Could you check a few things on this model? Use its own coordinates, in mm. A direction names the side the tool comes from. Coordinates: 2 decimals unless noted, no trailing zeros. Loops run counter-clockwise (first coordinate to the right, second up) from the corner with the lowest first, then second, coordinate; pieces in that order, holes last. Notation, with made-up numbers: M -35,-17 L -15,-17 A17 ccw -15,-9 Z; hole C 62.25,-32.5 d4. An arc over 180 degrees is marked long. Write each question's results on one line, items separated by ' | '.
```python
from build123d import *

# Parameters (mm, degrees)
F0_R     = 12.7
F1_DEPTH = 25.4
F2_R     = 15.875
F2_R_2   = 12.7
F3_DEPTH = 3.175


with BuildPart() as f1:
    # F0 (on Front) → F1 (new body)
    with BuildSketch(Plane.XZ):
        Circle(F0_R)
        with BuildLine():
            ThreePointArc((-1.8139228208, -1.778), (-0.9602697629, 2.351485059), (2.54, 0))
            ThreePointArc((2.54, 0), (2.351485059, -0.9602697629), (1.8139228208, -1.778))
            ThreePointArc((1.8139228208, -1.778), (0, -2.54), (-1.8139228208, -1.778))
        make_face(mode=Mode.SUBTRACT)
        with BuildLine():
            Line((1.8139228208, -1.778), (-1.8139228208, -1.778))
            ThreePointArc((-1.8139228208, -1.778), (0, -2.54), (1.8139228208, -1.778))
        make_face()
    extrude(amount=F1_DEPTH)

    # F2 (on face) → F3 (join)
    with BuildSketch(Plane.XZ.offset(25.4)):
        Circle(F2_R)
        Circle(F2_R_2, mode=Mode.SUBTRACT)
    extrude(amount=-F3_DEPTH)

    # F5: F1 across plane


with BuildPart() as f1_1:
    add(f1.part)
    add(f1.part.mirror(Plane(origin=(0, -12.7, -0.0066463366), x_dir=(1, 0, 0), z_dir=(0, 1, 0))))


solid = f1_1.part
```
(1) If we mould it in two halves opening along Y, with no side actions, what happens to faces 3 (the flat face through (3, 0, 0)), 4 (the flat face through (0, -13, -1.778)), 5 (the flat face through (-7, -3.175, 11))? For each: released by +Y, released by -Y, zero draft, split by the parting line, or undercut.
Reported:
face 3: released by +Y | face 4: zero draft | face 5: undercut
(2) Which directions (+Z, -Z, +X, -X, +Y, -Y) give clear straight access to the entire face, cutting with the end or side of a thin tool? Please do faces 1 (the cylindrical face through (-2.75, -12.57, -12.4)), 2 (the cylindrical face through (-3.441, -23.835, -15.497)).
Reported:
face 1: none | face 2: +Y, -Y
(3) Imagine slicing it at D-D, the plane z = -3. List the corners of the cut face in (x, y) for me (3 decimals), and give its area (3 significant figures).
Reported:
outline: M -15.589,-25.4 L 15.589,-25.4 L 15.589,-22.225 L 12.341,-22.225 L 12.341,-3.175 L 15.589,-3.175 L 15.589,0 L -15.589,0 L -15.589,-3.175 L -12.341,-3.175 L -12.341,-22.225 L -15.589,-22.225 Z | area: 668 mm2
(4) Will these pins go through, and if not, where does the flat tip stop? P1, Ø4, axis at y = -11.5, z = -0.5, coming from the +X side; P2, Ø2, axis at y = -21, z = -10, coming from the +X side; P3, Ø2, axis at x = -4, y = -9, coming from the +Z side.
Reported:
P1: stops at x = 12.7 | P2: stops at x = 8.96 | P3: stops at z = 12.34
(5) Please list where these lines run through material, in increasing order: probe 1 along Z at (x, y) = (0, -7); probe 2 along Y at (x, z) = (-13, 3) (3 decimals); probe 3 along X at (y, z) = (-14.75, -6). Write a range as from..to.
Reported:
probe 1: z = -12.7..-1.78, 2.54..12.7 | probe 2: y = -25.4..-22.225, -3.175..0 | probe 3: x = -11.19..11.19
(6) Imagine slicing it at A-A, the plane x = 0. List the corners of the cut face in (y, z) for me (3 decimals).
Reported:
outline: M -25.4,-15.875 L -22.225,-15.875 L -22.225,-12.7 L -3.175,-12.7 L -3.175,-15.875 L 0,-15.875 L 0,-1.778 L -25.4,-1.778 Z; M -25.4,2.54 L 0,2.54 L 0,15.875 L -3.175,15.875 L -3.175,12.7 L -22.225,12.7 L -22.225,15.875 L -25.4,15.875 Z
(7) Imagine slicing it at C-C, the plane y = -10.25. List the corners of the cut face in (x, z) for me, and give its area (3 significant figures).
Reported:
outline: C 0,0 d25.4; hole M -1.81,-1.78 L 1.81,-1.78 A2.54 ccw long Z | area: 488 mm2
(8) Imagine slicing it at B-B, the plane z = -14. List the corners of the cut face in (x, y) for me (3 decimals), and give its area (3 significant figures).
Reported:
outline: M -7.484,-25.4 L 7.484,-25.4 L 7.484,-22.225 L -7.484,-22.225 Z; M -7.484,-3.175 L 7.484,-3.175 L 7.484,0 L -7.484,0 Z | area: 95.1 mm2
